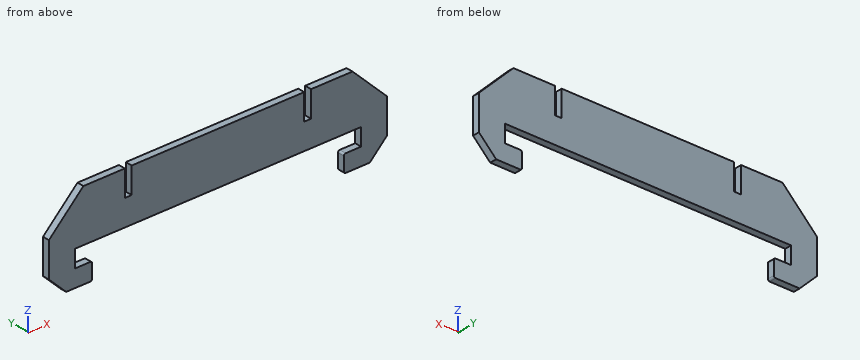
Autodesk Fusion 360 part; units mm, degrees
sketch "スケッチ1" plane through (0, 0, 0) normal (0, 1, 0) x (1, 0, 0)
  line L0 (98, 0) -> (98, 50)
  line L1 (98, 50) -> (73, 50)
  line L2 (73, 50) -> (73, 40)
  line L3 (73, 40) -> (83, 40)
  line L4 (83, 40) -> (83, 30)
  line L5 (83, 30) -> (-83, 30)
  line L6 (-83, 30) -> (-83, 40)
  line L7 (-83, 40) -> (-73, 40)
  line L8 (-73, 40) -> (-73, 50)
  line L9 (-73, 50) -> (-98, 50)
  line L10 (-98, 50) -> (-98, 0)
  line L11 (-98, 0) -> (-54, 0)
  line L12 (-54, 0) -> (-54, 15)
  line L13 (-54, 15) -> (-50, 15)
  line L14 (-50, 15) -> (-50, 0)
  line L15 (-50, 0) -> (50, 0)
  line L16 (50, 0) -> (50, 15)
  line L17 (50, 15) -> (54, 15)
  line L18 (54, 15) -> (54, 0)
  line L19 (54, 0) -> (98, 0)
  line L20 (-45, 20) -> (45, 20)
  point P0 (0, 30)
  dimension "d1" = 50
  dimension "d3" = 10
  dimension "d4" = 15
  dimension "d5" = 10
  dimension "d6" = 50
  dimension "d7" = 4
  dimension "d8" = 15
  dimension "d9" = 166
  dimension "d10" = 10
  dimension "d16" = 5
  dimension "d17" = 5
  dimension "d23" = 10
extrude "押し出し1" add sketch "スケッチ1" along normal blind 4
chamfer "面取り1" distance 20 angle 45 2 edges at (98, 2, 0) (-98, 2, 0)
chamfer "面取り2" distance 10 angle 45 2 edges at (98, 2, -50) (-98, 2, -50)
hole "穴1" at (0, 0, 0) at (0, 0, 0) direction (0, -1, 0) diameter 3.2 depth 4 tip angle 118
fillet "フィレット1" radius 1 4 edges at (-73, 2, -40) (73, 2, -40) (73, 2, -50) (-73, 2, -50)
Read the model definition and answer for the solid it produces. Units are mm, in the model's axes. Coordinates: 2 decimals unless noted, no trailing zeros. Loops run counter-clockwise (first coordinate to the right, second up) from the corner with the lowest first, then second, coordinate; pieces in that order, holes last. Notation, with made-up numbers: (64.5, 43.5) -> (91.5, 43.5) arc R29 ccw to (91.5, 70.5) -> close; hole circle Ø3 at (-15, -21.5). An arc over 180 degrees is marked (long way). Return JSON: item names as keys, results as strings.
Item 1: Find section D-D (y = 0.65). Determine the outline of the cut face in (x, z).
Answers:
{"outline": "(-98, -40) -> (-88, -50) -> (-74, -50) arc R1 ccw to (-73, -49) -> (-73, -41) arc R1 ccw to (-74, -40) -> (-83, -40) -> (-83, -30) -> (83, -30) -> (83, -40) -> (74, -40) arc R1 ccw to (73, -41) -> (73, -49) arc R1 ccw to (74, -50) -> (88, -50) -> (98, -40) -> (98, -20) -> (78, 0) -> (54, 0) -> (54, -15) -> (50, -15) -> (50, 0) -> (-50, 0) -> (-50, -15) -> (-54, -15) -> (-54, 0) -> (-78, 0) -> (-98, -20) -> close"}
Item 2: Flat-ended cylindrical pins translate along their axes: P1, Ø2, axis at x = -78.5, y = 3, coming from the +Z side; P2, Ø2, axis at y = 2, z = -9.5, coming from the -X side; P3, Ø2, axis at y = 1.5, z = -7.5, coming from the +X side; P4, Ø1.2, axis at y = 1.5, z = -46, coming from the +X side. Find the tip coordinate at first contact, or state that the pin passes through.
Answers:
{"P1": "stops at z = 0", "P2": "stops at x = -88.5", "P3": "stops at x = 86.5", "P4": "stops at x = 92.6"}
Item 3: Find the intervals of material crossed by probe 1 along X at (y, z) = (3.15, -35); probe 2 along X at (y, z) = (0.85, -11.5); probe 3 along Z at (x, y) = (77.5, 3.2), in increasing order.
Answers:
{"probe 1": "x = -98 to -83, 83 to 98", "probe 2": "x = -89.5 to -54, -50 to 50, 54 to 89.5", "probe 3": "z = -50 to -40, -30 to 0"}
Item 4: Find section C-C (z = -33.5). Determine the outline of the cut face in (x, y).
Answers:
{"outline": "(-98, 0) -> (-83, 0) -> (-83, 4) -> (-98, 4) -> close; (83, 0) -> (98, 0) -> (98, 4) -> (83, 4) -> close"}
Item 5: Find section B-B (x = 80). Determine the outline of the cut face in (y, z), plus the area to 3 significant figures.
Answers:
{"outline": "(0, -50) -> (4, -50) -> (4, -40) -> (0, -40) -> close; (0, -30) -> (4, -30) -> (4, -2) -> (0, -2) -> close", "area": "152 mm2"}
Item 6: Find section A-A (z = -9). Determine the outline of the cut face in (x, y).
Answers:
{"outline": "(-87, 0) -> (-54, 0) -> (-54, 4) -> (-87, 4) -> close; (-50, 0) -> (50, 0) -> (50, 4) -> (-50, 4) -> close; (54, 0) -> (87, 0) -> (87, 4) -> (54, 4) -> close"}
